Geometry check sheet. Reference: the model listing, model coordinates, mm. Round coordinates to 2 decimals unless told otherwise and drop trailing zeros. Order: outer loops, then holes, each group sorted by start corner. A loop starts at its lowest first (then second) coordinate and runs counter-clockwise, first axis right, second up. Notation, with made-up numbers: M 49.5,31 L 83.5,31 A30 cw 83.5,66 Z; hole C -39.5,36 d2. An arc over 180 degrees is marked long. Answer as a JSON object with one key per item and string values. Group by question number.
```python
from build123d import *

# Parameters (mm, degrees)
SKETCH1_R           = 6
BOSS_EXTRUDE1_DEPTH = 19.5
SKETCH1_3_R         = 1
BOSS_EXTRUDE2_DEPTH = 7.2
CUT_EXTRUDE4_DEPTH  = 55
SKETCH2_R           = 0.75
BOSS_EXTRUDE3_DEPTH = 4


with BuildPart() as part:
    # Sketch1 → Boss-Extrude1 (new body)
    with BuildSketch(Plane.XY):
        Circle(SKETCH1_R)
    extrude(amount=BOSS_EXTRUDE1_DEPTH)

    # Sketch1<3> → Boss-Extrude2 (add)
    with BuildSketch(Plane.XY):
        Circle(SKETCH1_3_R)
    extrude(amount=-BOSS_EXTRUDE2_DEPTH)

    # Sketch1<6> → Cut-Extrude4 (cut)
    with BuildSketch(Plane.XY):
        Polygon((0, 3.624712615), (0.894290994, 11.509067598), (-2.470474832, 11.33660338), align=None)
        Polygon((4.664832155, 10.623613465), (7.488356813, 8.785380219), (2.130552619, 2.932454105), align=None)
        Polygon((10.01833181, 5.85276429), (11.222124851, 2.7059762), (3.447306552, 1.120097798), align=None)
        Polygon((11.545169224, -1.153641916), (10.669422621, -4.407018754), (3.447306552, -1.120097798), align=None)
        Polygon((8.662144401, -7.71939612), (6.04136359, -9.836682333), (2.130552619, -2.932454105), align=None)
        Polygon((2.470474832, -11.33660338), (-0.894290994, -11.509067598), (0, -3.624712615), align=None)
        Polygon((-4.664832155, -10.623613465), (-7.488356813, -8.785380219), (-2.130552619, -2.932454105), align=None)
        Polygon((-10.01833181, -5.85276429), (-11.222124851, -2.7059762), (-3.447306552, -1.120097798), align=None)
        Polygon((-11.545169224, 1.153641916), (-10.669422621, 4.407018754), (-3.447306552, 1.120097798), align=None)
        Polygon((-8.662144401, 7.71939612), (-6.04136359, 9.836682333), (-2.130552619, 2.932454105), align=None)
    extrude(amount=CUT_EXTRUDE4_DEPTH, mode=Mode.SUBTRACT)

    # Sketch2 → Boss-Extrude3 (add)
    with BuildSketch(Plane.XY.offset(19.5)):
        Circle(SKETCH2_R)
    extrude(amount=BOSS_EXTRUDE3_DEPTH)


solid = part.part
```
1) Sectioned sample at B-B (y = 0). Record the boundary of the cut face in (x, z), then the cut area to 3 significant figures.
2) Sectioned sample at C-C (z = -1). Record the boundary of the cut face in (x, y).
3) Sectioned sample at D-D (x = 4.75). Record the boundary of the cut face in (y, z), then the cut area to 3 significant figures.
4) Go/stop test with flat-tipped pins: P1, Ø6, axis at x = -4, z = 20, coming from the -Y side; P2, Ø1.5, axis at y = 2.5, z = 12, coming from the +X side; P3, Ø1, axis at y = 2, z = -3, coming from the +X side; P4, Ø1, axis at x = 2.5, y = 1.5, coming from the +Z side. Record where each tip stops, or that it passes through.
5) Sectioned sample at A-A (x = -4.5). Record the boundary of the cut face in (y, z).
6) Thickness scan on line 1 along Z through (x, y) = (-4.5, -0.25); line 2 along X through (y, z) = (-3.5, 13); line 3 along Y through (x, z) = (-4, 13). Record the ranges inside material, lowest first. Write a range as [from, to].
7) Release check for a two-part mould opening along X. For faces 1 (the flat face through (4.63, 1.36, 9.61)), 2 (the cylindrical face through (1.64, 5.77, 9.61)), 3 (the flat face through (0, 0, 23.5)) record: +X half, -X half, draft (parallel to the pull), parting line (faces both ways), or undercut.
Final values:
{
 "1": {"outline": "M -6,0 L -1,0 L -1,-7.2 L 1,-7.2 L 1,0 L 6,0 L 6,19.5 L 0.75,19.5 L 0.75,23.5 L -0.75,23.5 L -0.75,19.5 L -6,19.5 Z", "area": "254 mm^2"},
 "2": {"outline": "C 0,0 d2"},
 "3": {"outline": "M -3.67,0 L -1.71,0 L -1.71,19.5 L -3.67,19.5 Z; M -1.13,0 L 1.39,0 L 1.39,19.5 L -1.13,19.5 Z; M 2.06,0 L 3.67,0 L 3.67,19.5 L 2.06,19.5 Z", "area": "118 mm^2"},
 "4": {"P1": "stops at y = -5.91", "P2": "stops at x = 5.43", "P3": "passes through", "P4": "stops at z = 19.5"},
 "5": {"outline": "M -3.97,0 L -1.88,0 L -1.88,19.5 L -3.97,19.5 Z; M -1.33,0 L 1.12,0 L 1.12,19.5 L -1.33,19.5 Z; M 1.6,0 L 3.97,0 L 3.97,19.5 L 1.6,19.5 Z"},
 "6": {"line 1": "z = [0, 19.5]", "line 2": "x = [-4.87, -2.65], [-2.32, 2.45], [2.9, 4.87]", "line 3": "y = [-4.47, -1.52], [-1.23, 1.12], [1.37, 4.3]"},
 "7": {"face 1": "undercut", "face 2": "+X half", "face 3": "draft"}
}
